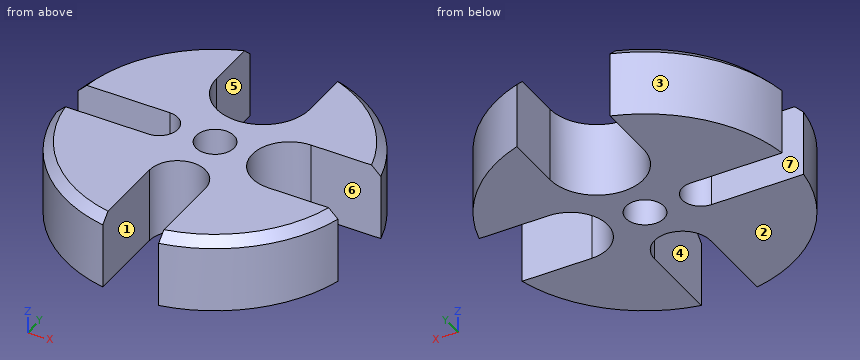
Autodesk Inventor part; units mm, degrees
ref_plane "YZ Plane" through (0, 0, 0) normal (1, 0, 0) x (0, 1, 0)
ref_plane "XZ Plane" through (0, 0, 0) normal (0, 1, 0) x (-1, 0, 0)
ref_plane "XY Plane" through (0, 0, 0) normal (0, 0, 1) x (1, 0, 0)
sketch "Sketch1" plane through (0, 0, 0) normal (0, 0, 1) x (1, 0, 0)
  line L0 (4.7625, 0) -> (6.35, 0)
  line L1 (0, -3.175) -> (0, -3.2385)
  arc A0 (12.7, 6.35) -> (12.7, -6.35) centre (12.7, 0) ccw
  arc A1 (-7.9502, 14.2748) -> (7.9502, 14.2748) centre (0, 14.2748) ccw
  arc A2 (-9.525, -3.175) -> (-9.525, 3.175) centre (-9.525, 0) ccw
  arc A3 (4.7625, -11.0998) -> (-4.7625, -11.0998) centre (0, -11.0998) ccw
  circle A4 centre (0, 0) radius 3.2385
  line L2 (7.9502, 14.2748) -> (7.9502, 24.1237)
  line L3 (-7.9502, 14.2748) -> (-7.9502, 24.1237)
  line L4 (12.7, 6.35) -> (24.5934, 6.35)
  line L5 (12.7, -6.35) -> (24.5934, -6.35)
  arc A5 (24.5934, 6.35) -> (7.9502, 24.1237) centre (0, 0) ccw
  line L6 (-9.525, 3.175) -> (-25.2008, 3.175)
  line L7 (-9.525, -3.175) -> (-25.2008, -3.175)
  arc A6 (-7.9502, 24.1237) -> (-25.2008, 3.175) centre (0, 0) ccw
  line L8 (-4.7625, -11.0998) -> (-4.7625, -24.9495)
  line L9 (4.7625, -11.0998) -> (4.7625, -24.9495)
  arc A7 (-25.2008, -3.175) -> (-4.7625, -24.9495) centre (0, 0) ccw
  arc A8 (4.7625, -24.9495) -> (24.5934, -6.35) centre (0, 0) ccw
  dimension "d5" = 6.477
  dimension "d1" = 12.7
  dimension "d2" = 15.9004
  dimension "d3" = 6.35
  dimension "d4" = 9.525
  dimension "d6" = 11.0998
  dimension "d7" = 14.2748
  dimension "d8" = 12.7
  dimension "d9" = 9.525
extrude "Extrusion1" add sketch "Sketch1" along normal blind 12.7
chamfer "Chamfer2" distance 1.524 angle 45 4 edges at (-19.6076, 16.1462, 12.7) (18.5405, 17.3612, 12.7) (17.3761, -18.5265, 12.7) (-18.5198, -17.3833, 12.7)
properties part number "Table" material "Stainless Steel"
CAD build for the part. Positions are in the model's coordinates, mm. Face numbers are marked on the shaded views. A direction names the side the tool comes from. Coordinates: 2 decimals unless noted, no trailing zeros. Write each loop counter-clockwise with the first axis right and the second up, starting at its lowest first coordinate (ties: lowest second). Pieces come first, ordered by that corner, then holes. Notation, with made-up numbers: (12.5, 14) -> (64.5, 14) arc R20 cw to (64.5, 26) -> close; hole circle Ø8 at (68.5, 6). An arc over 180 degrees is marked (long way). Return JSON: item names as keys, results as strings. Group by question number.
Q1. Which spindle directions (+Z, -Z, +X, -X, +Y, -Y) get a long thin tool onto all of the face, cutting with end or side? Do the marked faces 4, 5, 6 and 7. Say none if no direction does.
Q2. Cut at C-C, the plane y = 0. Give the cut face in (x, z).
Q3. Cut at A-A, the plane x = 0. Give the cut face in (y, z), then the cut area to 3 significant figures.
Q4. Pull direction X, two halves, no side cores. Call the marked faces 1, 2 and 3: released by +X, released by -X, zero draft, split by the parting line, or undercut.
Q5. Flat gauge pins, fed straight in: pin 1 (4 mm diameter, centred on x = 10.5, z = 5, fed in from +Y); pin 2 (1 mm diameter, centred on x = -12, z = 10, fed in from -Y); pin 3 (4 mm diameter, centred on x = -14.5, z = 9, fed in from +Y). Where does each tip first touch, or does it go through?
Q6. Drill centre lines: line 1 (Y direction, x = 0, z = 3.75); line 2 (X direction, y = 0, z = 8.5); line 3 (X direction, y = 20.5, z = 8). Where is each one in solid material? Low to high.
Returned:
{
 "1": {"face 4": "+Z, -Z, -Y", "face 5": "+Z, -Z, +Y", "face 6": "+Z, -Z, +X", "face 7": "+Z, -Z, -X"},
 "2": {"outline": "(-6.35, 0) -> (-3.24, 0) -> (-3.24, 12.7) -> (-6.35, 12.7) -> close; (3.24, 0) -> (6.35, 0) -> (6.35, 12.7) -> (3.24, 12.7) -> close"},
 "3": {"outline": "(-6.34, 0) -> (-3.24, 0) -> (-3.24, 12.7) -> (-6.34, 12.7) -> close; (3.24, 0) -> (6.32, 0) -> (6.32, 12.7) -> (3.24, 12.7) -> close", "area": "78.5 mm2"},
 "4": {"face 1": "undercut", "face 2": "zero draft", "face 3": "released by -X"},
 "5": {"pin 1": "stops at y = 23.94", "pin 2": "stops at y = -22.65", "pin 3": "stops at y = 22.11"},
 "6": {"line 1": "y = -6.34 to -3.24, 3.24 to 6.32", "line 2": "x = -6.35 to -3.24, 3.24 to 6.35", "line 3": "x = -15 to -7.95, 7.95 to 15"}
}
